Autodesk Inventor part; units mm, degrees
ref_plane "YZ Plane" through (0, 0, 0) normal (1, 0, 0) x (0, 1, 0)
ref_plane "XZ Plane" through (0, 0, 0) normal (0, 1, 0) x (-1, 0, 0)
ref_plane "XY Plane" through (0, 0, 0) normal (0, 0, 1) x (1, 0, 0)
sketch "Sketch1" plane through (0, 0, 0) normal (0, 1, 0) x (-1, 0, 0)
  line L0 (0, 0) -> (0, 39)
  line L1 (0, 39) -> (-28.713, 39)
  line L2 (-28.713, 39) -> (-28.713, 0)
  line L3 (-28.713, 0) -> (0, 0)
  dimension "d0" = 39
  dimension "d1" = 28.713
extrude "Extrusion1" add sketch "Sketch1" along normal blind 15
sketch "Sketch2" plane through (28.713, 0, 0) normal (0, 0, -1) x (-1, 0, 0)
  line L0 (28.713, 0) -> (28.713, 15)
  line L1 (0, 0) -> (28.713, 0)
  line L2 (2, 12) -> (26.713, 12)
  line L3 (2, 5.0411) -> (4.5, 5.0411)
  line L4 (4.5, 5.0411) -> (4.5, 2.0411)
  line L5 (4.5, 2.0411) -> (6, 2.0411)
  line L6 (6, 2.0411) -> (6, 0.5411)
  line L7 (6, 0.5411) -> (19.8539, 0.5411)
  line L8 (26.713, 5.0411) -> (24.213, 5.0411)
  line L9 (24.213, 5.0411) -> (24.213, 2.0411)
  line L10 (24.213, 2.0411) -> (22.713, 2.0411)
  line L11 (22.713, 2.0411) -> (22.713, 0.5411)
  line L12 (22.713, 0.5411) -> (19.8539, 0.5411)
  line L13 (2, 12) -> (2, 5.0411)
  line L14 (26.713, 12) -> (26.713, 5.0411)
  point P0 (0, 15)
  dimension "d7" = 2.5
  dimension "d8" = 3
  dimension "d9" = 1.5
  dimension "d10" = 1.5
  dimension "d11" = 2.5
  dimension "d12" = 3
  dimension "d13" = 1.5
  dimension "d14" = 1.5
extrude "Extrusion2" cut sketch "Sketch2" against normal blind 35
sketch "Sketch3" plane through (28.713, 0, 39) normal (1, 0, 0) x (0, 0, -1)
  line L0 (25.0019, 6.616) -> (0, 6.616)
  line L1 (0, 0) -> (0, 15)
  line L2 (25.0019, 6.616) -> (29.9465, 15)
  line L3 (0, 15) -> (39, 15)
  line L4 (29.9465, 15) -> (0, 15)
  line L5 (0, 6.616) -> (0, 15)
  point P0 (39, 0)
extrude "Extrusion3" cut sketch "Sketch3" against normal blind 0.5
chamfer "Chamfer1" distance 0.2 angle 45 1 edges at (28.713, 10.808, 11.5258)
sketch "Sketch4" plane through (0, 0, 0) normal (-1, 0, 0) x (0, 0, 1)
  line L0 (13.9981, 6.616) -> (39, 6.616)
  line L1 (39, 6.616) -> (13.9981, 6.616)
  line L2 (9.0535, 15) -> (13.9981, 6.616)
  line L3 (13.9981, 6.616) -> (9.0535, 15)
  line L4 (0, 15) -> (39, 15)
  line L5 (9.0535, 15) -> (39, 15)
  line L6 (39, 15) -> (39, 6.616)
  line L7 (39, 0) -> (39, 15)
  point P0 (0, 0)
extrude "Extrusion4" cut sketch "Sketch4" against normal blind 0.5
chamfer "Chamfer2" distance 0.5 angle 45 2 edges at (0.5, 15, 24.0267) (28.213, 15, 24.0267)
sketch "Sketch5" plane through (0, 15, 0) normal (0, 1, 0) x (1, 0, 0)
  line L0 (27.713, -9.0535) -> (27.713, -39)
  line L1 (27.713, -27.1604) -> (19.4998, -12.8142)
  line L2 (19.4998, -12.8142) -> (11.8392, -12.8142)
  line L3 (27.713, -39) -> (28.213, -39)
  line L4 (27.713, -27.1604) -> (27.713, -39)
  line L5 (1, -39) -> (27.713, -39)
  line L6 (27.713, -39) -> (1, -39)
  line L7 (1, -39) -> (1, -27.1604)
  line L8 (1, -39) -> (1, -9.0535)
  line L9 (1, -27.1604) -> (11.8392, -12.8142)
  point P0 (0, 0)
extrude "Extrusion5" cut sketch "Sketch5" against normal blind 0.2
properties part number "Port 1"
Can you work these out from the model? Positions are in its coordinate system, mm. A direction names the side the tool comes from. Round coordinates to 2 decimals unless told otherwise and drop trailing zeros. Write each loop counter-clockwise with the first axis right and the second up, starting at its lowest first coordinate (ties: lowest second). Pieces come first, ordered by that corner, then holes. Notation, with made-up numbers: M 16.25,8.25 L 75.25,8.25 A31 cw 75.25,45.25 Z; hole C -33,16 d11. An arc over 180 degrees is marked long. Use CSV: the item, a comma, the result in double quotes.
(1) I need wall thicknesses on line 1 along Y through (x, z) = (14, 16.5); line 2 along Y through (x, z) = (22.75, 2); line 3 along X through (y, z) = (4.25, 23). Which ranges of each line are inside material? Lowest first, please.
Check values:
line 1,"0 to 0.54, 12 to 14.8"
line 2,"0 to 2.04, 12 to 15"
line 3,"0 to 4.5, 24.21 to 28.71"
(2) Imagine slicing it at D-D (z = 16.5). Write out the boundary of the cut face in (x, y).
Check values:
outline,"M 0,0 L 28.71,0 L 28.71,6.62 L 28.21,6.62 L 28.21,14.5 L 27.71,15 L 21.61,15 L 21.61,14.8 L 9.05,14.8 L 9.05,15 L 1,15 L 0.5,14.5 L 0.5,6.62 L 0,6.62 Z; hole M 2,5.04 L 4.5,5.04 L 4.5,2.04 L 6,2.04 L 6,0.54 L 22.71,0.54 L 22.71,2.04 L 24.21,2.04 L 24.21,5.04 L 26.71,5.04 L 26.71,12 L 2,12 Z"
(3) Imagine slicing it at B-B (y = 1.5). Write out the boundary of the cut face in (x, z).
Check values:
outline,"M 0,0 L 6,0 L 6,35 L 22.71,35 L 22.71,0 L 28.71,0 L 28.71,39 L 0,39 Z"
(4) Imagine slicing it at C-C (x = 15.75). Write out the boundary of the cut face in (y, z).
Check values:
outline,"M 0,0 L 0.54,0 L 0.54,35 L 12,35 L 12,0 L 15,0 L 15,12.81 L 14.8,12.81 L 14.8,39 L 0,39 Z"
(5) Imagine slicing it at A-A (z = 33). Write out the boundary of the cut face in (x, y), plus the area to 3 significant figures.
Check values:
outline,"M 0,0 L 28.71,0 L 28.71,6.62 L 28.21,6.62 L 28.21,14.5 L 27.71,15 L 27.71,14.8 L 1,14.8 L 1,15 L 0.5,14.5 L 0.5,6.62 L 0,6.62 Z; hole M 2,5.04 L 4.5,5.04 L 4.5,2.04 L 6,2.04 L 6,0.54 L 22.71,0.54 L 22.71,2.04 L 24.21,2.04 L 24.21,5.04 L 26.71,5.04 L 26.71,12 L 2,12 Z"
area,"161 mm^2"
(6) On a 3-axis mill with a long thin cutter (end or side, diameter ignored), from which of +Z, -Z, +X, -X, +Y, -Y can I reach the whole of each face in a straight line? I mean faces 5 (the flat face through (0.5, 11, 24)), 6 (the flat face through (26.713, 9, 17)), 7 (the flat face through (0, 6, 15)). Say none if no direction works.
Check values:
face 5,"+Z, -X, +Y"
face 6,"-Z"
face 7,"+Z, -Z, -X, +Y, -Y"
(7) We'd pull the mould along Y, two halves only. Please class faces 1 (the flat face through (28.213, 11, 24)), 2 (the flat face through (14, 14.8, 29)), 3 (the flat face through (2, 9, 17)), 4 (the flat face through (15, 6, 35)): +Y half, -Y half, draft (parallel to the pull), parting line (faces both ways), or undercut.
Check values:
face 1,"draft"
face 2,"+Y half"
face 3,"undercut"
face 4,"undercut"
(8) I'm going to push flat-ended pins straight in: pin 1 (5 mm diameter, centred on x = 15.5, z = 24.5, fed in from +Y); pin 2 (3 mm diameter, centred on y = 12, z = 29.5, fed in from -X). Where does each tip first touch, or does it pass through?
Check values:
pin 1,"y = 14.8"
pin 2,"x = 0.5"
